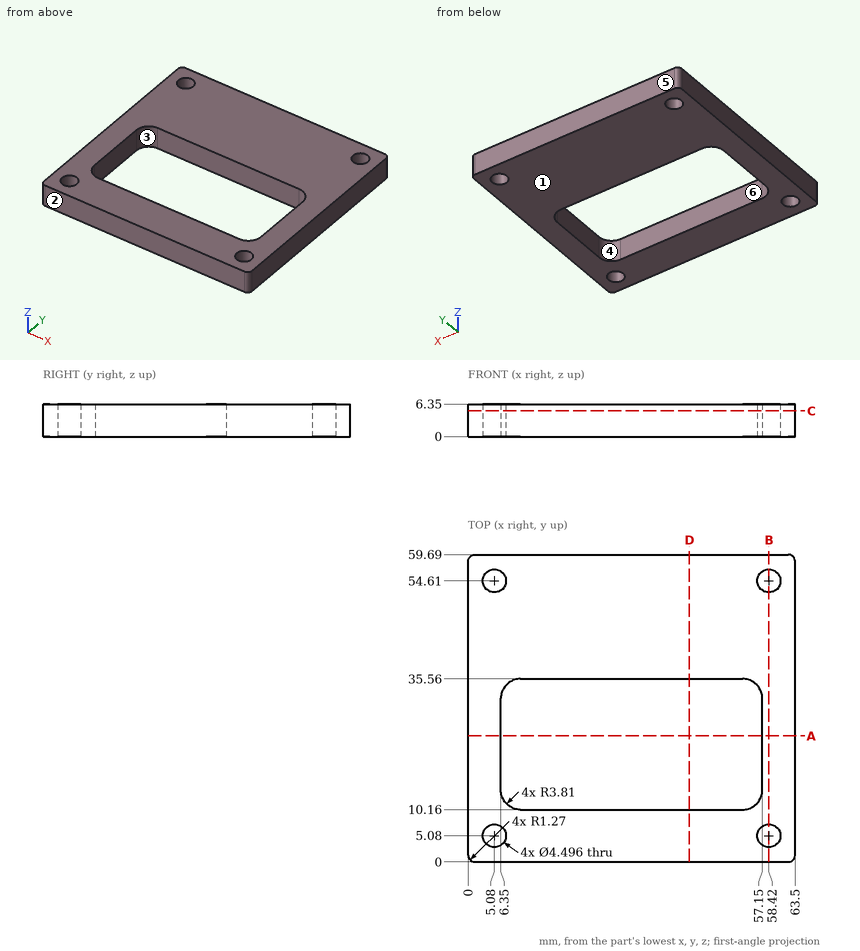
Geometry check sheet. Reference: drawing and pictorial views, mm from the part's lowest x, y, z. A direction names the side the tool comes from. Give positions to 0.01 mm unless a question says otherwise; leave off trailing zeros. Write each loop counter-clockwise with the first axis right and the second up, starting at its lowest first coordinate (ties: lowest second). Pieces come first, ordered by that corner, then holes.
Item 1: Access from +Z, -Z, +X, -X, +Y, -Y to the whole of each face (thin tool, end or side, straight path). Record for the marked faces 5 and 6.
Item 2: Gauge pin test, flat end, axial feed: pin 1 (2.5 mm diameter, centred on x = 5.08, y = 5.08, fed in from +Z). Record the tip position at first contact, or that the pin passes through.
Item 3: Cross-section at A-A (y = 24.5). Enter the section's corners in (x, z).
Item 4: Cross-section at B-B (x = 58.42). Enter the section's corners in (y, z).
Item 5: Cross-section at D-D (x = 43). Enter the section's corners in (y, z).
Item 6: Cross-section at C-C (z = 5). Enter the section's corners in (x, y).
Item 7: Draft check along Y on the marked faces 1, 2, 3 and 4. Enter one of: released by +Y, released by -Y, zero draft, split by the parting line, or undercut.
Item 8: Scan lines: L1, parallel to Y at x = 5.08, z = 2.5; L2, parallel to X at y = 5, z = 6.25; L3, parallel to Y at x = 34.5, z = 3.25. Record each from-to range of solid material in increasing order.
Report:
1. face 5: +Z, -Z, +X, -X, +Y
1. face 6: +Z, -Z
2. pin 1: passes through
3. outline: (0, 0) - (6.35, 0) - (6.35, 6.35) - (0, 6.35) - close; (57.15, 0) - (63.5, 0) - (63.5, 6.35) - (57.15, 6.35) - close
4. outline: (0, 0) - (2.83, 0) - (2.83, 6.35) - (0, 6.35) - close; (7.33, 0) - (52.36, 0) - (52.36, 6.35) - (7.33, 6.35) - close; (56.86, 0) - (59.69, 0) - (59.69, 6.35) - (56.86, 6.35) - close
5. outline: (0, 0) - (10.16, 0) - (10.16, 6.35) - (0, 6.35) - close; (35.56, 0) - (59.69, 0) - (59.69, 6.35) - (35.56, 6.35) - close
6. outline: (0, 1.27) arc R1.27 ccw to (1.27, 0) - (62.23, 0) arc R1.27 ccw to (63.5, 1.27) - (63.5, 58.42) arc R1.27 ccw to (62.23, 59.69) - (1.27, 59.69) arc R1.27 ccw to (0, 58.42) - close; hole circle Ø4.5 at (5.08, 5.08); hole circle Ø4.5 at (5.08, 54.61); hole (6.35, 13.97) arc R3.81 ccw to (10.16, 10.16) - (53.34, 10.16) arc R3.81 ccw to (57.15, 13.97) - (57.15, 31.75) arc R3.81 ccw to (53.34, 35.56) - (10.16, 35.56) arc R3.81 ccw to (6.35, 31.75) - close; hole circle Ø4.5 at (58.42, 5.08); hole circle Ø4.5 at (58.42, 54.61)
7. face 1: zero draft
7. face 2: released by -Y
7. face 3: undercut
7. face 4: undercut
8. L1: y = 0 to 2.83, 7.33 to 52.36, 56.86 to 59.69
8. L2: x = 0 to 2.83, 7.33 to 56.17, 60.67 to 63.5
8. L3: y = 0 to 10.16, 35.56 to 59.69
